from build123d import *

# Parameters (mm, degrees)
F0_W           = 46
F0_H           = 80
F1_DEPTH       = 25
F4_DEPTH       = 60
F2_W           = 0.5
F2_H           = 4
F2_W_2         = 20.5
F5_DEPTH       = 46
F8_DEPTH       = 3.5
F10_DEPTH      = 0.4
F2_W_3         = 25
F11_DEPTH      = 81
F11_DEPTH_BACK = 127
F14_DEPTH      = 3.5


with BuildPart() as f1:
    # F0 (on Front) → F1 (new body)
    with BuildSketch(Plane.XZ):
        with Locations((-12.4670048244, -31.5567021806)):
            Rectangle(F0_W, F0_H)
    extrude(amount=F1_DEPTH)

    # F3 (on face) → F4 (join)
    with BuildSketch(Plane.XY.offset(8.4432978194)):
        Polygon((10.5329951756, -25), (10.5329951756, 0), (-3.2170048244, 0), (-3.2170048244, -5), (5.5329951756, -5), (5.5329951756, -20), (-30.4670048244, -20), (-30.4670048244, -5), (-21.7170048244, -5), (-21.7170048244, 0), (-35.4670048244, 0), (-35.4670048244, -25), align=None)
    extrude(amount=F4_DEPTH)

    # F2 (on face) → F5 (join)
    with BuildSketch(Plane(origin=(-35.4670048244, 0, 0), x_dir=(0, -1, 0), z_dir=(-1, 0, 0))):
        with Locations((-0.25, -69.5567021806)):
            Rectangle(F2_W, F2_H)
        with Locations((35.25, -69.5567021806)):
            Rectangle(F2_W_2, F2_H)
        Polygon((-100, -71.5567021806), (-0.5, -71.5567021806), (-0.5, -67.5567021806), (-70, -67.5567021806), (-100, -67.5567021806), align=None)
        Polygon((45.5, -67.5567021806), (45.5, -71.5567021806), (145, -71.5567021806), (145, -67.5567021806), (115, -67.5567021806), align=None)
    extrude(amount=-F5_DEPTH)

    # F7 (on offset) → F8 (join, symmetric)
    with BuildSketch(Plane(origin=(-12.4670048244, 0, 0), x_dir=(0, -1, 0), z_dir=(-1, 0, 0))):
        Polygon((0, -67.5567021806), (0, 2.4432978194), (-70, -67.5567021806), align=None)
        Polygon((25, 2.4432978194), (25, -67.5567021806), (115, -67.5567021806), align=None)
    extrude(amount=F8_DEPTH, both=True)

    # F10 (add, through all): a face of the model
    f10_faces = [f1.faces().sort_by_distance(p)[0] for p in [
        (-12.4670048244, -11.0375494071, 8.4432978194),
    ]]
    extrude(f10_faces, amount=F10_DEPTH)

    # F2 (on face) → F11 (join, two sides)
    with BuildSketch(Plane(origin=(-35.4670048244, 0, 0), x_dir=(0, -1, 0), z_dir=(-1, 0, 0))) as f11_sk:
        with Locations((-0.25, -69.5567021806)):
            Rectangle(F2_W, F2_H)
        with Locations((12.5, -69.5567021806)):
            Rectangle(F2_W_3, F2_H)
        with Locations((35.25, -69.5567021806)):
            Rectangle(F2_W_2, F2_H)
    extrude(amount=F11_DEPTH)
    extrude(f11_sk.sketch, amount=-F11_DEPTH_BACK)

    # F13 (on offset) → F14 (join, symmetric)
    with BuildSketch(Plane(origin=(0, -12.5, 0), x_dir=(-1, 0, 0), z_dir=(0, 1, 0))):
        Polygon((103.0237070051, -67.5567021806), (35.4670048244, 0), (-10.5329951756, 0), (-78.0896973562, -67.5567021806), align=None)
    extrude(amount=F14_DEPTH, both=True)


solid = f1.part
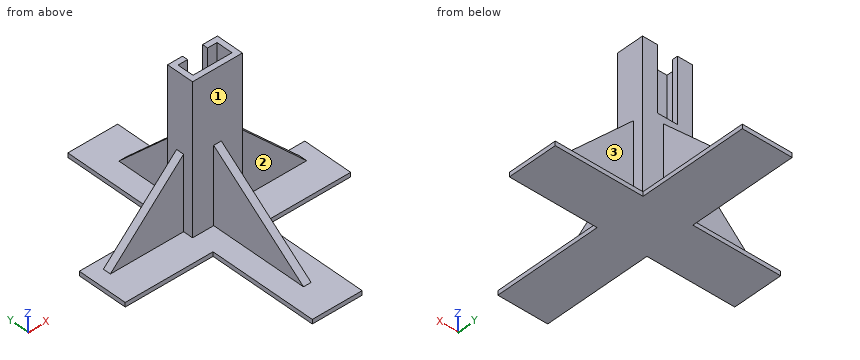
Work out the finished part from the listing and answer in its coordinate system (mm). Face numbers are marked on the shaded views. A direction names the side the tool comes from. Round coordinates to 2 decimals unless told otherwise and drop trailing zeros. Write each loop counter-clockwise with the first axis right and the second up, starting at its lowest first coordinate (ties: lowest second). Pieces come first, ordered by that corner, then holes.
1) Straight lines are drawn through the part: line 1 (X direction, y = -4, z = 53.5); line 2 (X direction, y = -75, z = -36.5); line 3 (Y direction, x = -9, z = 61). For each, find the intervals that lie inside material, in ascending order.
2) A tool of negligible diameter and unlimited length cuts with its end or side. For the marked faces 1, 2 and 3, from which of +Z, -Z, +X, -X, +Y, -Y can it reach the whole face along a straight path? Write none if from no direction.
3) A cutting plane is placed at B-B (x = 1.5). Give the vertices of the cut face in (y, z), plus the area to 3 significant figures.
4) A cutting plane is placed at C-C (y = -72). Give the vertices of the cut face in (x, z), plus the area to 3 significant figures.
5) Given pin 1 Ø6 at (x, z) = (-26, -45) entering from +Y; pin 2 Ø2 at (y, z) = (45.5, -70) entering from +X; pin 3 Ø1.5 at (y, z) = (-2.5, 34) entering from -X, each flat-ended and moving along its own axis, determine where each tip first touches the part or whether it passes through.
6) A cutting plane is placed at D-D (x = 25). Give the vertices of the cut face in (y, z).
7) A cutting plane is placed at A-A (z = 23.5). Give the vertices of the cut face in (x, y), plus the area to 4 significant figures.
Completed:
1. line 1: x = -35.47 to -21.72, -3.22 to 10.53
1. line 2: x = -15.97 to -8.97
1. line 3: y = -25 to -20
2. face 1: +Z, -Y
2. face 2: +Z, +X, -Y
2. face 3: +Z, +X, +Y
3. outline: (-145, -71.56) - (100, -71.56) - (100, -67.56) - (0, -67.56) - (0, 68.44) - (-5, 68.44) - (-5, 8.84) - (-20, 8.84) - (-20, 68.44) - (-25, 68.44) - (-25, -67.56) - (-145, -67.56) - close
3. area: 3,490 mm2
4. outline: (-35.47, -71.56) - (10.53, -71.56) - (10.53, -67.56) - (-8.97, -67.56) - (-8.97, -34.11) - (-15.97, -34.11) - (-15.97, -67.56) - (-35.47, -67.56) - close
4. area: 418 mm2
5. pin 1: stops at y = 0
5. pin 2: stops at x = 10.53
5. pin 3: stops at x = -35.47
6. outline: (-45.5, -71.56) - (0.5, -71.56) - (0.5, -67.56) - (-9, -67.56) - (-9, -14.47) - (-16, -14.47) - (-16, -67.56) - (-45.5, -67.56) - close
7. outline: (-35.47, -25) - (10.53, -25) - (10.53, 0) - (-3.22, 0) - (-3.22, -5) - (5.53, -5) - (5.53, -20) - (-30.47, -20) - (-30.47, -5) - (-21.72, -5) - (-21.72, 0) - (-35.47, 0) - close
7. area: 517.5 mm2
